Input: part model. Units: mm. Frame: model coordinates. A direction names the side the tool comes from. Round coordinates to 2 decimals unless told otherwise and drop trailing zeros. Write each loop counter-clockwise with the first axis right and the second up, starting at its lowest first coordinate (ties: lowest second). Pieces come first, ordered by that corner, then holes. Notation, with made-up numbers: M 17,-18 L 44,-18 A9 cw 44,-1 Z; hole C -10.5,40 d4. An arc over 180 degrees is marked long. Use one line per item in the form item = value. Start each with the question number.
```python
from build123d import *

# Parameters (mm, degrees)
SKETCH1_R           = 3
SKETCH1_R_2         = 2.5
BOSS_EXTRUDE1_DEPTH = 27.5
BOSS_EXTRUDE2_DEPTH = 4


with BuildPart() as part:
    # Sketch1 → Boss-Extrude1 (new body)
    with BuildSketch(Plane(origin=(0, 0, 0), x_dir=(1, 0, 0), z_dir=(0, 1, 0))):
        Circle(SKETCH1_R)
        Circle(SKETCH1_R_2, mode=Mode.SUBTRACT)
    extrude(amount=BOSS_EXTRUDE1_DEPTH)

    # Sketch2 → Boss-Extrude2 (add)
    with BuildSketch(Plane.XZ):
        Polygon((0, 5.773502692), (-5, 2.886751346), (-5, -2.886751346), (0, -5.773502692), (5, -2.886751346), (5, 2.886751346), align=None)
    extrude(amount=BOSS_EXTRUDE2_DEPTH)


solid = part.part
```
Item 1: First-contact query: pin 1 (3 mm diameter, centred on x = -0.5, z = -0.5, fed in from +Y); pin 2 (1.5 mm diameter, centred on x = 0, y = 18.5, fed in from -Z); pin 3 (4 mm diameter, centred on y = 6, z = -1.5, fed in from -X). Flat tips, straight axial feed; report the tip coordinate or a pass-through.
Item 2: Reachability of faces 1 (the face through (2.2, 0, -2.5)), 2 (the face through (-5, -2, 0)) from +Z, -Z, +X, -X, +Y, -Y: full face, straight path, thin tool, end or side. Return the list, or none.
Item 3: Ray query, line 1 (X direction, y = 17, z = 0); line 2 (Y direction, x = 1.75, z = -2.75). Return the intervals inside material, ascending. Write a range as from..to.
Item 4: Cut plane D-D (x = -3.5). Output: boundary loops of the cut face in (y, z).
Item 5: Cut plane A-A (x = -0.5). Output: boundary loops of the cut face in (y, z), plus the area to 3 significant figures.
Item 6: Draft query along X for faces 3 (the face through (2.535, -1.972, 4.31)), 4 (the face through (-0.54, 13.56, 2.44)), 5 (the face through (0, -4, 0)). Return one class per face: +X half, -X half, draft (parallel to the pull), parting line (faces both ways), or undercut.
Item 7: Cut plane B-B (z = -1.75). Output: boundary loops of the cut face in (x, y), plus the area to 3 significant figures.
Item 8: Cut plane C-C (y = 11.5). Output: boundary loops of the cut face in (x, z), plus the area to 3 significant figures.
Final values:
q1.pin_1 = 0
q1.pin_2 = -3
q1.pin_3 = -3
q2.face_1 = +Y
q2.face_2 = +Z, -Z, -X, +Y, -Y
q3.line_1 = -3..-2.5, 2.5..3
q3.line_2 = -4..0
q4.outline = M -4,-3.75 L 0,-3.75 L 0,3.75 L -4,3.75 Z
q5.outline = M -4,-5.48 L 0,-5.48 L 0,-2.96 L 27.5,-2.96 L 27.5,-2.45 L 0,-2.45 L 0,2.45 L 27.5,2.45 L 27.5,2.96 L 0,2.96 L 0,5.48 L -4,5.48 Z
q5.area = 71.8 mm^2
q6.face_3 = +X half
q6.face_4 = undercut
q6.face_5 = draft
q7.outline = M -5,-4 L 5,-4 L 5,0 L 2.44,0 L 2.44,27.5 L 1.79,27.5 L 1.79,0 L -1.79,0 L -1.79,27.5 L -2.44,27.5 L -2.44,0 L -5,0 Z
q7.area = 75.8 mm^2
q8.outline = C 0,0 d6; hole C 0,0 d5
q8.area = 8.64 mm^2
